Check sheet for the modelled part. Datum: model origin and axes. Units: mm. A direction names the side the tool comes from. Round coordinates to 2 decimals unless told otherwise and drop trailing zeros. Loops run counter-clockwise (first coordinate to the right, second up) from the corner with the lowest first, then second, coordinate; pieces in that order, holes last. Notation, with made-up numbers: (35, 14.5) -> (79, 14.5) arc R29 cw to (79, 41.5) -> close; hole circle Ø8 at (6, -10.75). An arc over 180 degrees is marked (long way). One line per item, written item: value. Start each with the question number.
1. Cross-section at C-C on y = -1. Record the cut outline in (x, z), then the cut area to 3 significant figures.
2. Cross-section at A-A on y = 2. Record the cut outline in (x, z).
3. Material ranges on L1, parallel to Y at x = 0, z = -8.5; L2, parallel to X at y = 3.5, z = -11.75; L3, parallel to X at y = 0.75, z = -4.75, recorded low to high.
4. Release check for a two-part mould opening along X. For faces 3 (the face through (-0.23, 9.98, -8.91)), 4 (the face through (-18.96, 6.24, -9.08)), 5 (the face through (-1.726, 5.045, -1.726)) record: +X half, -X half, draft (parallel to the pull), parting line (faces both ways), or undercut.
5. Set-up check for faces 1 (the face through (18.901, 6.313, -9.081)), 2 (the face through (1.8, 5, -1.7)): record each of +Z, -Z, +X, -X, +Y, -Y from which the full face is reachable in a straight line by a thin tool's end or side.
6. Cross-section at B-B on z = -12. Record the cut outline in (x, y), then the cut area to 3 significant figures.
7. Go/stop test with flat-tipped pins: pin 1 (2 mm diameter, centred on y = -5, z = -7, fed in from -X); pin 2 (2 mm diameter, centred on x = -12, z = -7.5, fed in from -Y); pin 3 (5 mm diameter, centred on x = -12, z = -12, fed in from +Y). Record where each tip stops, or that it passes through.
from build123d import *

# Parameters (mm, degrees)
F0_W     = 40
F0_H     = 20
F1_DEPTH = 15
F3_DEPTH = 3.5
F5_DEPTH = 15.001
F6_R     = 2
F7_DEPTH = 11.501
F8_R     = 5
F9_R     = 2.9936248173


with BuildPart() as f1:
    # F0 (on Top) → F1 (new body)
    with BuildSketch(Plane.XY):
        Rectangle(F0_W, F0_H)
    extrude(amount=-F1_DEPTH)

    # F2 (on face) → F3 (cut)
    with BuildSketch(Plane.XY):
        Polygon((3.5, -0.0207259422), (3.5, 4.0207259422), (0, 6.0414518843), (-3.5, 4.0207259422), (-3.5, -0.0207259422), (0, -2.0414518843), align=None)
    extrude(amount=-F3_DEPTH, mode=Mode.SUBTRACT)

    # F4 (on face) → F5 (cut, through all)
    with BuildSketch(Plane.XY):
        with BuildLine():
            ThreePointArc((-20, 7), (0, 9.9805733622), (20, 7))
            Line((20, 7), (20, 10))
            Line((20, 10), (-20, 10))
            Line((-20, 10), (-20, 7))
        make_face()
        with BuildLine():
            Line((-20, -10), (20, -10))
            ThreePointArc((20, -10), (0, -7.0601321922), (-20, -10))
        make_face()
    extrude(amount=-F5_DEPTH, mode=Mode.SUBTRACT)

    # F6 (on face) → F7 (cut, through all)
    with BuildSketch(Plane.XY.offset(-3.5)):
        with Locations((0, 2)):
            Circle(F6_R)
    extrude(amount=-F7_DEPTH, mode=Mode.SUBTRACT)

    # F8
    f8_edges = [f1.edges().sort_by_distance(p)[0] for p in [
        (-20, 7, -7.5),
        (20, 7, -7.5),
        (-20, -10, -7.5),
        (20, -10, -7.5),
    ]]
    fillet(f8_edges, radius=F8_R)

    # F9
    f9_edges = [f1.edges().sort_by_distance(p)[0] for p in [
        (0, 9.980573, 0),
        (-20, -0.199833, 0),
        (20, -0.199833, 0),
        (0, -7.060132, 0),
    ]]
    fillet(f9_edges, radius=F9_R)


solid = f1.part
Taken from the geometry:
1. outline: (-20, -15) -> (20, -15) -> (20, -2.99) arc R2.99 ccw to (17.01, 0) -> (1.8, 0) -> (1.8, -3.5) -> (-1.8, -3.5) -> (-1.8, 0) -> (-17.01, 0) arc R2.99 ccw to (-20, -2.99) -> close
1. area: 584 mm2
2. outline: (-20, -15) -> (-2, -15) -> (-2, -3.5) -> (-3.5, -3.5) -> (-3.5, 0) -> (-17.01, 0) arc R2.99 ccw to (-20, -2.99) -> close; (2, -15) -> (20, -15) -> (20, -2.99) arc R2.99 ccw to (17.01, 0) -> (3.5, 0) -> (3.5, -3.5) -> (2, -3.5) -> close
3. L1: y = -7.06 to 0, 4 to 9.98
3. L2: x = -19.99 to -1.32, 1.32 to 19.99
3. L3: x = -20 to -1.56, 1.56 to 20
4. face 3: parting line
4. face 4: -X half
4. face 5: undercut
5. face 1: +Z, -Z, +X, +Y
5. face 2: +Z
6. outline: (-20, -3.59) arc R5 ccw to (-13.99, -8.48) arc R69.5 cw to (13.99, -8.48) arc R5 ccw to (20, -3.59) -> (20, 3.19) arc R5 ccw to (16.18, 8.05) arc R68.59 ccw to (-16.18, 8.05) arc R5 ccw to (-20, 3.19) -> close; hole circle Ø4 at (0, 2)
6. area: 645 mm2
7. pin 1: stops at x = -19.98
7. pin 2: stops at y = -8.29
7. pin 3: stops at y = 9.32
